```python
from build123d import *

# Parameters (mm, degrees)
CYLINDER001_R     = 12.5
CYLINDER001_DEPTH = 24
CYLINDER002_R     = 13.5
CYLINDER002_DEPTH = 13
CYLINDER_R        = 17
CYLINDER_DEPTH    = 8
CYLINDER003_R     = 11.5
CYLINDER003_DEPTH = 25
CYLINDER004_R     = 18
CYLINDER004_DEPTH = 14


with BuildPart() as innerhole:
    # Cylinder001 → Cylinder001 (new body)
    with BuildSketch(Plane.XY.offset(-5)):
        Circle(CYLINDER001_R)
    extrude(amount=CYLINDER001_DEPTH)


with BuildPart() as sleeve:
    # Cylinder002 → Cylinder002 (new body)
    with BuildSketch(Plane.XY):
        Circle(CYLINDER002_R)
    extrude(amount=CYLINDER002_DEPTH)


with BuildPart() as cut:
    # Cylinder → Cylinder (new body)
    with BuildSketch(Plane.XY):
        Circle(CYLINDER_R)
    extrude(amount=CYLINDER_DEPTH)

    # Fusion: union Sleeve
    add(sleeve.part)

    # Cut: cut InnerHole
    add(innerhole.part, mode=Mode.SUBTRACT)


with BuildPart() as materialsaving:
    # Cylinder003 → Cylinder003 (new body)
    with BuildSketch(Plane.XY):
        Circle(CYLINDER003_R)
    extrude(amount=CYLINDER003_DEPTH)


with BuildPart() as cut002:
    # Cylinder004 → Cylinder004 (new body)
    with BuildSketch(Plane.XY):
        Circle(CYLINDER004_R)
    extrude(amount=CYLINDER004_DEPTH)

    # Cut001: cut MaterialSaving
    add(materialsaving.part, mode=Mode.SUBTRACT)

    # Cut002: cut Cut
    add(cut.part, mode=Mode.SUBTRACT)


solid = cut002.part
```
Can you work these out from the model? Positions are in its coordinate system, mm. A direction names the side the tool comes from. Coordinates: 2 decimals unless noted, no trailing zeros. Loops run counter-clockwise (first coordinate to the right, second up) from the corner with the lowest first, then second, coordinate; pieces in that order, holes last.
1) Which directions (+Z, -Z, +X, -X, +Y, -Y) give clear straight access to the entire face, cutting with the end or side of a thin tool? Please do faces 4 (the cylindrical face through (11.923, 3.755, 6.409)), 5 (the flat face through (16, -7, 0)).
2) Thinking about a two-plate mould opening in Y: for faces 1 (the cylindrical face through (-2.343, 17.847, 6.902)), 2 (the cylindrical face through (9.139, 14.334, 3.944)), 3 (the flat face through (11, -4, 0)), which applies, pulls with the +Y half, pulls with the -Y half, needs draft (parallel to the pull), parting line crosses it, or undercut?
3) I need wall thicknesses on probe 1 along Y at (x, z) = (0, 4); probe 2 along Y at (x, z) = (1.5, 0.75); probe 3 along X at (y, z) = (7, 9.5). Which ranges of each line are inside material? Lowest first, please.
4) Imagine slicing it at C-C on z = 1.5. List the corners of the cut face in (x, y) for me.
5) For pin 1 (2 mm diameter, centred on y = 1.5, z = 6, fed in from -X); pin 2 (2 mm diameter, centred on y = -10, z = 8, fed in from +X); pin 3 (3 mm diameter, centred on x = 13.5, z = 11, fed in from -Y), each with a flat end and sliding along its axis, tell me the tip position at first contact or that it passes through.
6) Imagine slicing it at D-D on y = -14. List the corners of the cut face in (x, z) for me, plus the area to 3 significant figures.
7) Imagine slicing it at A-A on y = 0. List the corners of the cut face in (x, z) for me, plus the area to 4 significant figures.
Completed:
1. face 4: -Z
1. face 5: -Z, +X, -X, +Y, -Y
2. face 1: parting line crosses it
2. face 2: undercut
2. face 3: needs draft
3. probe 1: y = -18 to -17, -12.5 to -11.5, 11.5 to 12.5, 17 to 18
3. probe 2: y = -17.94 to -16.93, -12.41 to -11.4, 11.4 to 12.41, 16.93 to 17.94
3. probe 3: x = -16.58 to -11.54, -10.36 to -9.12, 9.12 to 10.36, 11.54 to 16.58
4. outline: circle Ø36 at (0, 0); circle Ø25 at (0, 0); hole circle Ø34 at (0, 0); hole circle Ø23 at (0, 0)
5. pin 1: stops at x = -17.99
5. pin 2: stops at x = 15.59
5. pin 3: stops at y = -13.42
6. outline: (-11.31, 0) - (-9.64, 0) - (-9.64, 8) - (9.64, 8) - (9.64, 0) - (11.31, 0) - (11.31, 14) - (-11.31, 14) - close
6. area: 162 mm2
7. outline: (-18, 0) - (-17, 0) - (-17, 8) - (-13.5, 8) - (-13.5, 13) - (-12.5, 13) - (-12.5, 0) - (-11.5, 0) - (-11.5, 14) - (-18, 14) - close; (11.5, 0) - (12.5, 0) - (12.5, 13) - (13.5, 13) - (13.5, 8) - (17, 8) - (17, 0) - (18, 0) - (18, 14) - (11.5, 14) - close
7. area: 100.0 mm2
